```python
from build123d import *

# Parameters (mm, degrees)
SKETCH_1_W          = 43.5396
SKETCH_1_H          = 45
SKETCH_1_W_2        = 5
SKETCH_1_H_2        = 3.1
EXTRUDE_1_DEPTH     = 3.4
SKETCH_2_W          = 43.6316
SKETCH_2_H          = 45
SKETCH_2_RX         = 1
SKETCH_2_RY         = 1
SKETCH_2_W_2        = 5.2
SKETCH_2_H_2        = 5.2
EXTRUDE_2_DEPTH     = 1
SKETCH_6_W          = 0.092
SKETCH_6_H          = 1
CUT_EXTRUDE_2_DEPTH = 46
SKETCH_3_R          = 4
SKETCH_3_R_2        = 1
EXTRUDE_3_DEPTH     = 1.2
SKETCH_4_W          = 43.5396
SKETCH_4_H          = 45
SKETCH_4_W_2        = 39.5596
SKETCH_4_H_2        = 41.02
EXTRUDE_4_DEPTH     = 5
SKETCH_5_W          = 1.99
SKETCH_5_H          = 25
CUT_EXTRUDE_1_DEPTH = 5


with BuildPart() as part:
    # Эскиз1 → Бобышка-Вытянуть1 (new body)
    with BuildSketch(Plane(origin=(0, 0, 0), x_dir=(1, 0, 0), z_dir=(0, 1, 0))):
        with Locations((-126.7302, -82.5)):
            Rectangle(SKETCH_1_W, SKETCH_1_H)
        with Locations((-141, -96.2003)):
            Rectangle(SKETCH_1_W_2, SKETCH_1_H_2, mode=Mode.SUBTRACT)
        with Locations((-118.4, -96.2003)):
            Rectangle(SKETCH_1_W_2, SKETCH_1_H_2, mode=Mode.SUBTRACT)
        with Locations((-112.2, -93.2003)):
            Rectangle(SKETCH_1_W_2, SKETCH_1_H_2, mode=Mode.SUBTRACT)
        with Locations((-134.8, -93.2003)):
            Rectangle(SKETCH_1_W_2, SKETCH_1_H_2, mode=Mode.SUBTRACT)
        with Locations((-112.2, -87.1003)):
            Rectangle(SKETCH_1_W_2, SKETCH_1_H_2, mode=Mode.SUBTRACT)
        with Locations((-134.8, -87.1003)):
            Rectangle(SKETCH_1_W_2, SKETCH_1_H_2, mode=Mode.SUBTRACT)
        with Locations((-141, -90.1003)):
            Rectangle(SKETCH_1_W_2, SKETCH_1_H_2, mode=Mode.SUBTRACT)
        with Locations((-118.4, -90.1003)):
            Rectangle(SKETCH_1_W_2, SKETCH_1_H_2, mode=Mode.SUBTRACT)
        with Locations((-112.2, -74.9003)):
            Rectangle(SKETCH_1_W_2, SKETCH_1_H_2, mode=Mode.SUBTRACT)
        with Locations((-134.8, -74.9003)):
            Rectangle(SKETCH_1_W_2, SKETCH_1_H_2, mode=Mode.SUBTRACT)
        with Locations((-141, -77.9003)):
            Rectangle(SKETCH_1_W_2, SKETCH_1_H_2, mode=Mode.SUBTRACT)
        with Locations((-118.4, -77.9003)):
            Rectangle(SKETCH_1_W_2, SKETCH_1_H_2, mode=Mode.SUBTRACT)
        with Locations((-141, -84.0003)):
            Rectangle(SKETCH_1_W_2, SKETCH_1_H_2, mode=Mode.SUBTRACT)
        with Locations((-118.4, -84.0003)):
            Rectangle(SKETCH_1_W_2, SKETCH_1_H_2, mode=Mode.SUBTRACT)
        with Locations((-112.2, -81.0003)):
            Rectangle(SKETCH_1_W_2, SKETCH_1_H_2, mode=Mode.SUBTRACT)
        with Locations((-134.8, -81.0003)):
            Rectangle(SKETCH_1_W_2, SKETCH_1_H_2, mode=Mode.SUBTRACT)
        with Locations((-141, -71.8003)):
            Rectangle(SKETCH_1_W_2, SKETCH_1_H_2, mode=Mode.SUBTRACT)
        with Locations((-118.4, -71.8003)):
            Rectangle(SKETCH_1_W_2, SKETCH_1_H_2, mode=Mode.SUBTRACT)
        with Locations((-112.2, -68.8003)):
            Rectangle(SKETCH_1_W_2, SKETCH_1_H_2, mode=Mode.SUBTRACT)
        with Locations((-134.8, -68.8003)):
            Rectangle(SKETCH_1_W_2, SKETCH_1_H_2, mode=Mode.SUBTRACT)
    extrude(amount=EXTRUDE_1_DEPTH)

    # Эскиз2 → Бобышка-Вытянуть2 (add)
    with BuildSketch(Plane(origin=(0, 0, 0), x_dir=(1, 0, 0), z_dir=(0, 1, 0))):
        with Locations((-126.6842, -82.5)):
            Rectangle(SKETCH_2_W, SKETCH_2_H)
        with Locations(Location((-143.5, -65), (0, 0, 180))):
            Ellipse(SKETCH_2_RX, SKETCH_2_RY, mode=Mode.SUBTRACT)
        with Locations(Location((-143.5, -100), (0, 0, 180))):
            Ellipse(SKETCH_2_RX, SKETCH_2_RY, mode=Mode.SUBTRACT)
        with Locations(Location((-109.7, -65), (0, 0, 180))):
            Ellipse(SKETCH_2_RX, SKETCH_2_RY, mode=Mode.SUBTRACT)
        with Locations(Location((-109.7, -100), (0, 0, 180))):
            Ellipse(SKETCH_2_RX, SKETCH_2_RY, mode=Mode.SUBTRACT)
        with Locations((-134.8, -68.8)):
            Rectangle(SKETCH_2_W_2, SKETCH_2_H_2, mode=Mode.SUBTRACT)
        with Locations((-134.8, -74.9)):
            Rectangle(SKETCH_2_W_2, SKETCH_2_H_2, mode=Mode.SUBTRACT)
        with Locations((-134.8, -81)):
            Rectangle(SKETCH_2_W_2, SKETCH_2_H_2, mode=Mode.SUBTRACT)
        with Locations((-134.8, -87.1)):
            Rectangle(SKETCH_2_W_2, SKETCH_2_H_2, mode=Mode.SUBTRACT)
        with Locations((-134.8, -93.2003)):
            Rectangle(SKETCH_2_W_2, SKETCH_2_H_2, mode=Mode.SUBTRACT)
        with Locations((-118.4, -71.8003)):
            Rectangle(SKETCH_2_W_2, SKETCH_2_H_2, mode=Mode.SUBTRACT)
        with Locations((-118.4, -77.9003)):
            Rectangle(SKETCH_2_W_2, SKETCH_2_H_2, mode=Mode.SUBTRACT)
        with Locations((-118.4, -84.0003)):
            Rectangle(SKETCH_2_W_2, SKETCH_2_H_2, mode=Mode.SUBTRACT)
        with Locations((-118.4, -90.1003)):
            Rectangle(SKETCH_2_W_2, SKETCH_2_H_2, mode=Mode.SUBTRACT)
        with Locations((-118.4, -96.2003)):
            Rectangle(SKETCH_2_W_2, SKETCH_2_H_2, mode=Mode.SUBTRACT)
    extrude(amount=-EXTRUDE_2_DEPTH)

    # Эскиз6 → Вырез-Вытянуть2 (cut, through all)
    with BuildSketch(Plane(origin=(0, 0, 60), x_dir=(-1, 0, 0), z_dir=(0, 0, -1))):
        with Locations((104.9144, -0.5)):
            Rectangle(SKETCH_6_W, SKETCH_6_H)
    extrude(amount=-CUT_EXTRUDE_2_DEPTH, mode=Mode.SUBTRACT)

    # Эскиз3 → Бобышка-Вытянуть3 (add)
    with BuildSketch(Plane.XZ.offset(1)):
        with Locations((-143.5, 100)):
            Circle(SKETCH_3_R)
        with Locations((-143.5, 100)):
            Circle(SKETCH_3_R_2, mode=Mode.SUBTRACT)
        with Locations((-109.7, 100)):
            Circle(SKETCH_3_R)
        with Locations((-109.7, 100)):
            Circle(SKETCH_3_R_2, mode=Mode.SUBTRACT)
        with Locations((-143.5, 65)):
            Circle(SKETCH_3_R)
        with Locations((-143.5, 65)):
            Circle(SKETCH_3_R_2, mode=Mode.SUBTRACT)
        with Locations((-109.7, 65)):
            Circle(SKETCH_3_R)
        with Locations((-109.7, 65)):
            Circle(SKETCH_3_R_2, mode=Mode.SUBTRACT)
    extrude(amount=EXTRUDE_3_DEPTH)

    # Эскиз4 → Бобышка-Вытянуть4 (add)
    with BuildSketch(Plane.XZ.offset(1)):
        with Locations((-126.7302, 82.5)):
            Rectangle(SKETCH_4_W, SKETCH_4_H)
        with Locations((-126.7302, 82.5)):
            Rectangle(SKETCH_4_W_2, SKETCH_4_H_2, mode=Mode.SUBTRACT)
    extrude(amount=EXTRUDE_4_DEPTH)

    # Эскиз5 → Вырез-Вытянуть1 (cut)
    with BuildSketch(Plane.XZ.offset(6)):
        with Locations((-147.505, 82.5)):
            Rectangle(SKETCH_5_W, SKETCH_5_H)
        with Locations((-105.9554, 82.5)):
            Rectangle(SKETCH_5_W, SKETCH_5_H)
    extrude(amount=-CUT_EXTRUDE_1_DEPTH, mode=Mode.SUBTRACT)


solid = part.part
```
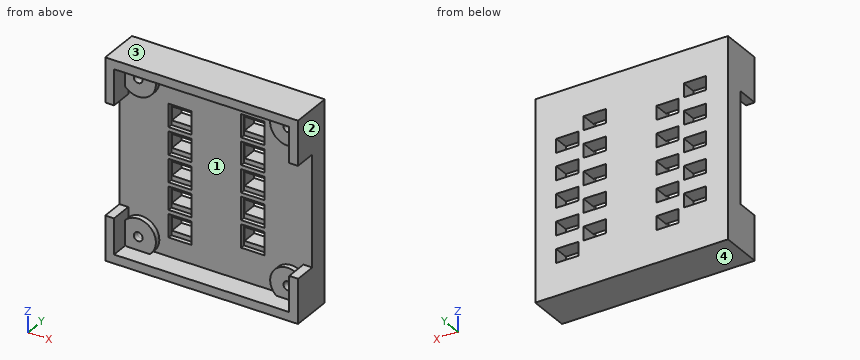
Input: part model. Units: mm. Frame: model coordinates. Face numbers are marked on the shaded views. Coordinates: 2 decimals unless noted, no trailing zeros. Loops run counter-clockwise (first coordinate to the right, second up) from the corner with the lowest first, then second, coordinate; pieces in that order, holes last. Notation, with made-up numbers: M 10,-22 L 44,-22 A9 cw 44,-17 Z; hole C 54,23.25 d1. An arc over 180 degrees is marked long. Use a Markdown table: item, result. Add a question column.
1) Section A-A, the plane y = -4.25. Return the cut outline in (x, z).
2) Draft query along Z for the marked faces 1, 2, 3 and 4. Return one class per face: +Z half, -Z half, draft (parallel to the pull), parting line (faces both ways), or undercut.
3) Section B-B, the plane x = -131. Return the cut outline in (y, z).
4) Section C-C, the plane x = -117. Give the number of separate pieces and of enclosed holes in the cut face, plus the area to 3 significant figures.
5) Line query: L1, parallel to Z at x = -143.5, y = -1.6; L2, parallel to X at y = -1.9, z = 100; L3, parallel to X at y = 0.75, z = 93.5. Output: solid intervals per line, ascending. Write a range as from..to.
6) Pin query (flat end, axial travel): P1, Ø1.6, axis at x = -143, z = 100, coming from the -Y side; P2, Ø8, axis at x = -131, z = 88.5, coming from the -Y side. Return the tip coordinate at first contact, or that it passes through.
Answer below:
| question | item | result |
|---|---|---|
| 1 | outline | M -148.5,60 L -104.96,60 L -104.96,70 L -106.95,70 L -106.95,61.99 L -146.51,61.99 L -146.51,70 L -148.5,70 Z; M -148.5,95 L -146.51,95 L -146.51,103.01 L -106.95,103.01 L -106.95,95 L -104.96,95 L -104.96,105 L -148.5,105 Z |
| 2 | face 1 | undercut |
| 2 | face 2 | draft |
| 2 | face 3 | +Z half |
| 2 | face 4 | -Z half |
| 3 | outline | M -6,60 L 3.4,60 L 3.4,105 L -6,105 L -6,103.01 L -1,103.01 L -1,61.99 L -6,61.99 Z |
| 4 | separate pieces | 6 |
| 4 | enclosed holes | 0 |
| 4 | area | 139 mm2 |
| 5 | L1 | 60..64, 66..69, 96..99, 101..105 |
| 5 | L2 | -148.5..-144.5, -142.5..-139.5, -113.7..-110.7, -108.7..-104.96 |
| 5 | L3 | -148.5..-137.3, -132.3..-114.7, -109.7..-104.96 |
| 6 | P1 | y = -2.2 |
| 6 | P2 | y = -1 |
